Verification items for the finished model (mm, model axes). A direction names the side the tool comes from. Coordinates: 2 decimals unless noted, no trailing zeros. Order: outer loops, then holes, each group sorted by start corner. A loop starts at its lowest first (then second) coordinate and runs counter-clockwise, first axis right, second up. Notation, with made-up numbers: M 11.5,8.5 L 36.5,8.5 A8 ccw 36.5,14.5 Z; hole C 8.25,63.5 d7. An arc over 180 degrees is marked long. Return JSON: item names as keys, results as strings. Group by question number.
Q1. Go/stop test with flat-tipped pins: pin 1 Ø2 at (y, z) = (2, -2) entering from -X; pin 2 Ø1.5 at (x, y) = (1.5, -0.5) entering from +Z (3 decimals); pin 3 Ø1 at (x, z) = (7, -1.5) entering from -Y. Record where each tip stops, or that it passes through.
Q2. Section check A-A, the plane x = 18.5. Enter the section's corners in (y, z) (3 decimals), then the cut area to 3 significant figures.
Q3. Mould release check, pull along Y, two halves, no side actions. Record for faces 3 (the face through (-4, 0.952, 0)), 4 (the face through (0, -2, 4)), 5 (the face through (-4, -0.952, 0)), 6 (the face through (-2.13, -1.03, 4.65)): pulls with the +Y half, pulls with the -Y half, needs draft (parallel to the pull), parting line crosses it, or undercut.
Q4. Access from +Z, -Z, +X, -X, +Y, -Y to the whole of each face (thin tool, end or side, straight path). Record for faces 1 (the face through (12.19, -0.69, 3.1)), 2 (the face through (-3.023, 0, 0)).
Q5. Thickness scan on probe 1 along Y at (x, z) = (1, 0) (3 decimals); probe 2 along Z at (x, y) = (-3.5, -1); probe 3 along Y at (x, z) = (12.5, -0.75). Record the ranges inside material, lowest first.
Autodesk Inventor part; units mm, degrees
ref_plane "IDS_WORKPLANE{1}" through (-5.4864, 0, 0) normal (1, 0, 0) x (0, 0, -1)
ref_plane "Work Plane2" through (41.275, 0, 0) normal (0, 0, -1) x (1, 0, 0)
ref_plane "YZ Plane" through (0, 0, 0) normal (1, 0, 0) x (0, 1, 0)
sketch "Szkic1" plane through (0, 0, 0) normal (0, 0, 1) x (1, 0, 0)
  line L0 (-5.4864, 0) -> (25.4, 0)
  line L1 (25.4, 0) -> (25.4, 3.175)
  line L2 (25.4, 3.175) -> (6.35, 3.175)
  line L3 (6.35, 3.175) -> (5.588, 3.175)
  line L4 (5.588, 3.175) -> (0, 3.175)
  line L5 (0, 3.175) -> (0, 4.7625)
  line L6 (-12.0399, 0) -> (31.64, 0)
  line L7 (0, -0.9693) -> (0, 5.8158)
  line L8 (0, 4.7625) -> (-4.2103, 4.7625)
  arc A0 (-4.2103, 4.7625) -> (-5.4864, 0) centre (4.0386, 0) ccw
  line L9 (6.35, 3.175) -> (0, 3.175) construction
  dimension "d0" = 25.4
  dimension "d1" = 19.05
  dimension "d2" = 0.762
  dimension "d3" = 5.4864
  dimension "d4" = 6.35
  dimension "d5" = 6.35
  dimension "d9" = 9.525
  dimension "d10" = 0
  dimension "d13" = 9.525
revolve "Bryła" add sketch "Szkic1" angle 360 about axis through (-5.4864, 0, 0) along (1, 0, 0)
ref_plane "IDS_WORKPLANE{1}" through (-5.4864, 0, 0) normal (1, 0, 0) x (0, 0, -1)
sketch "Szkic2" plane through (-5.4864, 0, 0) normal (1, 0, 0) x (0, 0, -1)
  circle A0 centre (0, 0) radius 4.7625
  line L0 (0, -6.6675) -> (0, 6.6675)
  line L1 (6.6675, 0) -> (-6.6675, 0)
  line L2 (-4.7625, 0.9525) -> (4.7625, 0.9525)
  line L3 (4.7625, 0.9525) -> (4.7625, -0.9525)
  line L4 (4.7625, -0.9525) -> (-4.7625, -0.9525)
  line L5 (-4.7625, -0.9525) -> (-4.7625, 0.9525)
  line L6 (-4.7625, 0) -> (4.7625, 0) construction
  line L7 (0, 0.9525) -> (0, -0.9525) construction
  dimension "d15" = 1.905
extrude "Szczelina" cut sketch "Szkic2" along normal blind 2.4638 contours L1 L0 L2 A0 | L3 L4 A0 | A0 L4 L0 L1 | A0 L2 L3 | L1 A0 L2 L0 | L0 L4 A0 L1 | L5 L2 A0 | A0 L4 L5
thread "Gwint"
sketch "Szkic3" plane through (0, 0, 0) normal (0, 0, 1) x (1, 0, 0)
  line L0 (25.4, 0) -> (25.4, 3.175)
  line L1 (25.4, 3.175) -> (6.35, 3.175)
  line L2 (-5.4864, 0) -> (25.4, 0)
  arc A0 (25.4, 0) -> (24.5493, 3.175) centre (19.05, 0) ccw
  line L3 (25.4, -3.175) -> (25.4, 3.175)
  line L4 (24.5493, 3.175) -> (24.5493, 0)
  line L5 (24.5493, 0) -> (25.4, 0)
  dimension "d40" = 6.35
revolve "Zaokrąglenie1" cut sketch "Szkic3" angle 360 about axis through (-5.4864, 0, 0) along (1, 0, 0) contours A0 L1 L0
chamfer "Faza" distance 0.635 angle 45 1 edges at (24.5493, -3.175, 0)
ref_plane "Work Plane2" through (41.275, 0, 0) normal (0, 0, -1) x (1, 0, 0)
fillet "Zaokrąglenie4" radius 0.7874 1 edges at (0, -3.175, 0)
equation "\"d0\" = NLG"
equation "\"d1\" = GEL"
equation "\"d2\" = GAL"
equation "\"d3\" = KOH"
equation "\"d4\" = GD"
equation "\"d5\" = BDM"
equation "\"d9\" = KOD"
equation "\"d13\" = KR"
equation "\"d15\" = SBR"
equation "\"d16\" = STI"
equation "\"d40\" = GD"
equation "\"d11\" = GEL"
equation "\"d43\" = 0.5 * RR"
equation "\"d46\" = R"
equation "\"GD\" = NND"
equation "\"NLG\" = 25.4"
equation "\"GEL\" = 19.05"
equation "\"KOD\" = 9.525"
equation "\"KOH\" = 5.4864"
equation "\"GAL\" = 0.762"
equation "\"BDM\" = NND"
equation "\"SBR\" = 1.905"
equation "\"STI\" = 2.4638"
equation "\"KEWI\" = 0"
equation "\"KR\" = KOD"
equation "\"d14\" = -KOH"
equation "\"R\" = 0.7874"
equation "\"THREADDIA\" = 6.35"
equation "\"TOA\" = 30deg"
equation "\"KOH1\" = 4.3688"
equation "\"NND\" = 6.35"
equation "\"GD1\" = 4.8387"
equation "\"THREADDESC\" = 1.2345"
properties part number "ANSI B18.6.2 - 1/4-20 UNC - 1" material "Stal, miękka"
Numbers:
{
 "1": {"pin 1": "stops at x = -5.31", "pin 2": "stops at z = 3.175", "pin 3": "stops at y = -3.01"},
 "2": {"outline": "C 0,0 d6.35", "area": "31.7 mm2"},
 "3": {"face 3": "undercut", "face 4": "needs draft", "face 5": "undercut", "face 6": "parting line crosses it"},
 "4": {"face 1": "+X", "face 2": "+Z, -Z, -X"},
 "5": {"probe 1": "y = -3.175 to 3.175", "probe 2": "z = -4.66 to 4.66", "probe 3": "y = -3.09 to 3.09"}
}
